The model under review builds one solid part; all positions refer to its coordinate system, in mm. A direction names the side the tool comes from. Round coordinates to 2 decimals unless told otherwise and drop trailing zeros. Write each loop counter-clockwise with the first axis right and the second up, starting at its lowest first coordinate (ties: lowest second). Pieces come first, ordered by that corner, then holes. Notation, with made-up numbers: (17.5, 77) -> (68.5, 77) arc R21 ccw to (68.5, 89) -> close; hole circle Ø2 at (52.25, 16.25). An arc over 180 degrees is marked (long way). Answer as a JSON object with one key per item and string values. Group by question number.
1) To check wall thickness, follow probe 1 along Z at (x, y) = (70, 22.5); probe 2 along X at (y, z) = (30.5, 93.5); probe 3 along X at (y, z) = (45.5, 92.5). State the ranges of each line that lie inside material, in increasing order. Write a range as [from, to].
2) We need section A-A, the plane z = -68. Write out the cut boundary in (x, y).
3) We need section C-C, the plane x = 32.5. Write out the cut boundary in (y, z).
4) Mouldability with a two-part tool opening along X and no side actions: class faces 4 (the flat face through (-109, 28, 1)), 5 (the flat face through (-2, 28, 103)), 6 (the flat face through (56, 31, -1)) as pulls with the +X half, pulls with the -X half, needs draft (parallel to the pull), parting line crosses it, or undercut.
5) Machinability: for faces 1 (the flat face through (-58, 2, -52)), 2 (the flat face through (-1, 57, 0)), 3 (the flat face through (-5, 48, -1)), which of the approach directions +Z, -Z, +X, -X, +Y, -Y give a long, thin tool a straight path to every point of the face, cutting with its end or side? Answer none if there is none.
6) We need section B-B, the plane y = 37.5. Write out the cut boundary in (x, z), then the cut area to 3 significant figures.
7) Insertion check: pin 1 Ø12 at (x, z) = (20, 34.5) entering from +Y; pin 2 Ø11 at (x, z) = (-0.5, -42) entering from -Y. Each pin has a flat end and moves straight along its axis. Give the tip position at first contact, or say it passes through.
from build123d import *

# Parameters (mm, degrees)
SKETCH1_W           = 218
SKETCH1_H           = 206
SKETCH1_W_2         = 100
SKETCH1_H_2         = 100
BOSS_EXTRUDE1_DEPTH = 57
SKETCH2_W           = 218
SKETCH2_H           = 206
BOSS_EXTRUDE2_DEPTH = 2
FILLET1_R           = 4
SKETCH3_W           = 10
SKETCH3_H           = 10
CUT_EXTRUDE1_DEPTH  = 240.929156211


with BuildPart() as part:
    # Sketch1 → Boss-Extrude1 (new body)
    with BuildSketch(Plane(origin=(0, 0, 0), x_dir=(1, 0, 0), z_dir=(0, 1, 0))):
        Rectangle(SKETCH1_W, SKETCH1_H)
        with Locations((-57, -51)):
            Rectangle(SKETCH1_W_2, SKETCH1_H_2, mode=Mode.SUBTRACT)
        with Locations((57, -51)):
            Rectangle(SKETCH1_W_2, SKETCH1_H_2, mode=Mode.SUBTRACT)
        with Locations((-57, 51)):
            Rectangle(SKETCH1_W_2, SKETCH1_H_2, mode=Mode.SUBTRACT)
        with Locations((57, 51)):
            Rectangle(SKETCH1_W_2, SKETCH1_H_2, mode=Mode.SUBTRACT)
    extrude(amount=BOSS_EXTRUDE1_DEPTH)

    # Sketch2 → Boss-Extrude2 (add)
    with BuildSketch(Plane(origin=(0, 0, 0), x_dir=(1, 0, 0), z_dir=(0, 1, 0))):
        Rectangle(SKETCH2_W, SKETCH2_H)
    extrude(amount=BOSS_EXTRUDE2_DEPTH)

    # Fillet1
    fillet1_edges = [part.edges().sort_by_distance(p)[0] for p in [
        (57, 2, -1),
        (-57, 2, 1),
        (-107, 2, 51),
        (-57, 2, 101),
        (-7, 2, 51),
        (57, 2, 1),
        (7, 2, 51),
        (57, 2, 101),
        (107, 2, 51),
        (-57, 2, -1),
        (-7, 2, -51),
        (-57, 2, -101),
        (-107, 2, -51),
        (107, 2, -51),
        (57, 2, -101),
        (7, 2, -51),
    ]]
    fillet(fillet1_edges, radius=FILLET1_R)

    # Sketch3 → Cut-Extrude1 (cut, through all)
    with BuildSketch(Plane(origin=(0, 0, -103), x_dir=(-1, 0, 0), z_dir=(0, 0, -1))):
        with Locations((0, 48)):
            Rectangle(SKETCH3_W, SKETCH3_H)
    extrude(amount=-CUT_EXTRUDE1_DEPTH, mode=Mode.SUBTRACT)


solid = part.part
Here are the results:
{
 "1": {"probe 1": "z = [-103, -101], [-1, 1], [101, 103]", "probe 2": "x = [-109, -107], [-7, 7], [107, 109]", "probe 3": "x = [-109, -107], [-7, -5], [5, 7], [107, 109]"},
 "2": {"outline": "(-109, 0) -> (109, 0) -> (109, 57) -> (107, 57) -> (107, 6) arc R4 cw to (103, 2) -> (11, 2) arc R4 cw to (7, 6) -> (7, 57) -> (-7, 57) -> (-7, 6) arc R4 cw to (-11, 2) -> (-103, 2) arc R4 cw to (-107, 6) -> (-107, 57) -> (-109, 57) -> close; hole (-5, 43) -> (5, 43) -> (5, 53) -> (-5, 53) -> close"},
 "3": {"outline": "(0, -103) -> (57, -103) -> (57, -101) -> (6, -101) arc R4 cw to (2, -97) -> (2, -5) arc R4 cw to (6, -1) -> (57, -1) -> (57, 1) -> (6, 1) arc R4 cw to (2, 5) -> (2, 97) arc R4 cw to (6, 101) -> (57, 101) -> (57, 103) -> (0, 103) -> close"},
 "4": {"face 4": "pulls with the -X half", "face 5": "needs draft", "face 6": "undercut"},
 "5": {"face 1": "+Y", "face 2": "+Z, -Z, +X, -X, +Y", "face 3": "+Z, -Z"},
 "6": {"outline": "(-109, -103) -> (109, -103) -> (109, 103) -> (-109, 103) -> close; hole (-107, -101) -> (-7, -101) -> (-7, -1) -> (-107, -1) -> close; hole (-107, 1) -> (-7, 1) -> (-7, 101) -> (-107, 101) -> close; hole (7, -101) -> (107, -101) -> (107, -1) -> (7, -1) -> close; hole (7, 1) -> (107, 1) -> (107, 101) -> (7, 101) -> close", "area": "4,910 mm^2"},
 "7": {"pin 1": "stops at y = 2", "pin 2": "stops at y = 0"}
}
